Geometry: see drawing. Coordinates: mm, zero at the bounding-box minimum. A direction names the side the tool comes from. Give positions to 0.01 mm unless a question says otherwise; leave off trailing zeros. Order: outer loops, then holes, each group sorted by start corner. A loop starts at its lowest first (then second) coordinate and runs counter-clockwise, first axis right, second up. Notation, with made-up numbers: (42.25, 19.25) -> (62.25, 19.25) arc R23 cw to (62.25, 42.25) -> close; hole circle Ø2 at (88.25, -35.5). An arc over 180 degrees is marked (long way). One line per item, written item: value. Start each with the question number.
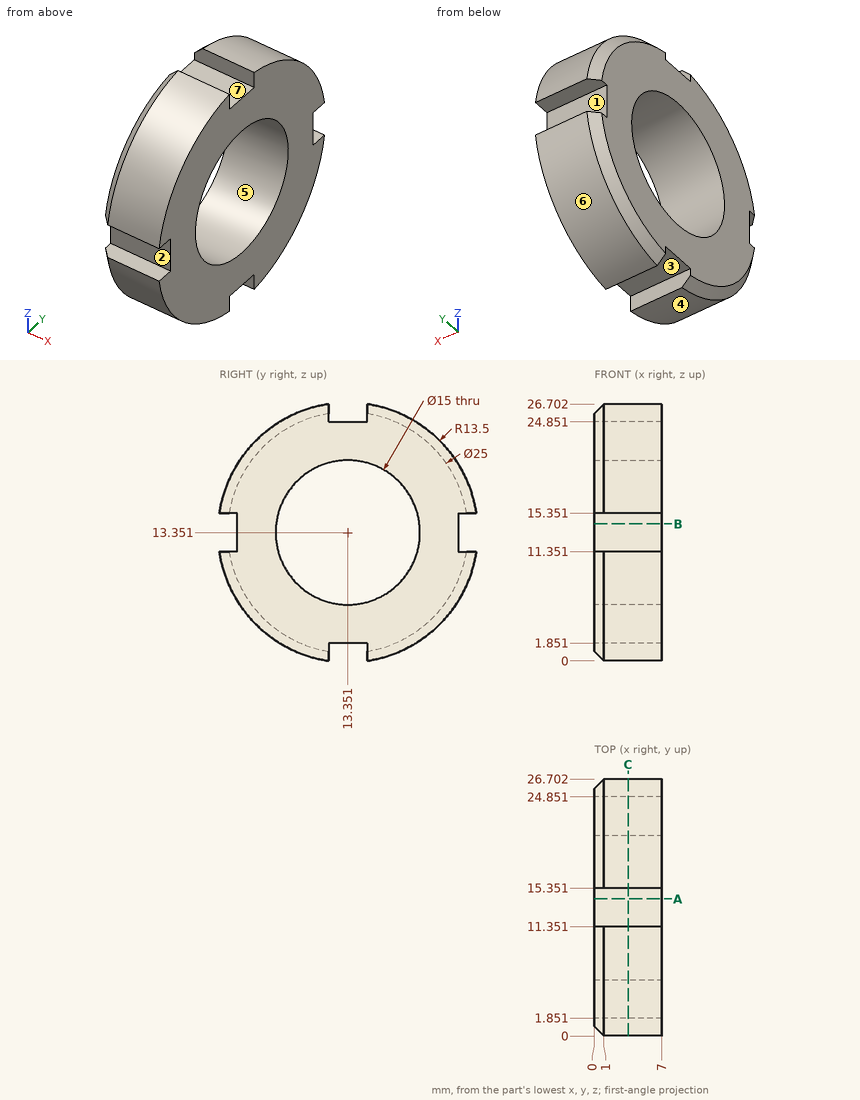
1. Cut plane C-C, the plane x = 3.5. Return loops of the section in (y, z), then the cut area to 3 significant figures.
2. Material intervals for L1, parallel to Z at x = 6.5, y = 18.75 (1 decimal); L2, parallel to Y at x = 2.25, z = 12; L3, parallel to Z at x = 6.5, y = 10, sorted ascending. Write a range as [from, to].
3. Pin query (flat end, axial travel): P1, Ø0.9, axis at x = 2, z = 0.5, coming from the +Y side; P2, Ø1.5, axis at x = 4.5, y = 1, coming from the +Z side (3 decimals); P3, Ø4, axis at x = 3.5, y = 5, coming from the -Z side. Return the tip coordinate at first contact, or that it passes through.
4. Cut plane A-A, the plane y = 14.25. Return loops of the section in (x, z) (3 decimals).
5. Draft query along Y for the marked faces 4, 5, 6 and 7. Return one class per face: pulls with the +Y half, pulls with the -Y half, needs draft (parallel to the pull), parting line crosses it, or undercut.
6. Access query for the marked faces 1, 2 and 3. Directions: +Z, -Z, +X, -X, +Y, -Y. A direction counts if a zero-diameter tool reaches every point of the face in a straight line with its end or side. Return the directions, or none.
Answers follow:
1. outline: (0, 11.35) arc R13.5 ccw to (11.35, 0) -> (11.35, 1.85) -> (15.35, 1.85) -> (15.35, 0) arc R13.5 ccw to (26.7, 11.35) -> (24.85, 11.35) -> (24.85, 15.35) -> (26.7, 15.35) arc R13.5 ccw to (15.35, 26.7) -> (15.35, 24.85) -> (11.35, 24.85) -> (11.35, 26.7) arc R13.5 ccw to (0, 15.35) -> (1.85, 15.35) -> (1.85, 11.35) -> close; hole circle Ø15 at (13.35, 13.35)
1. area: 365 mm²
2. L1: z = [1, 8.1], [18.6, 25.7]
2. L2: y = [1.85, 5.97], [20.73, 24.85]
2. L3: z = [0.27, 6.64], [20.06, 26.43]
3. P1: stops at y = 18.69
3. P2: stops at z = 20.255
3. P3: stops at z = 1.44
4. outline: (0, 1.851) -> (7, 1.851) -> (7, 5.905) -> (0, 5.905) -> close; (0, 20.797) -> (7, 20.797) -> (7, 24.851) -> (0, 24.851) -> close
5. face 4: pulls with the -Y half
5. face 5: undercut
5. face 6: pulls with the +Y half
5. face 7: undercut
6. face 1: +X, -X, +Y
6. face 2: +X, -X, -Y
6. face 3: -Z, +X, -X
